Source: three-view drawing plus pictorial views. Frame: mm from the lowest corner of the part. A direction names the side the tool comes from. Coordinates: 2 decimals unless noted, no trailing zeros. Write each loop counter-clockwise with the first axis right and the second up, starting at its lowest first coordinate (ties: lowest second). Pieces come first, ordered by that corner, then holes. Notation, with made-up numbers: (24, -32) - (60, -32) arc R14 cw to (60, -7) - close; hole circle Ø1 at (57, 2). An arc over 180 degrees is marked (long way). One line per item, written item: value.
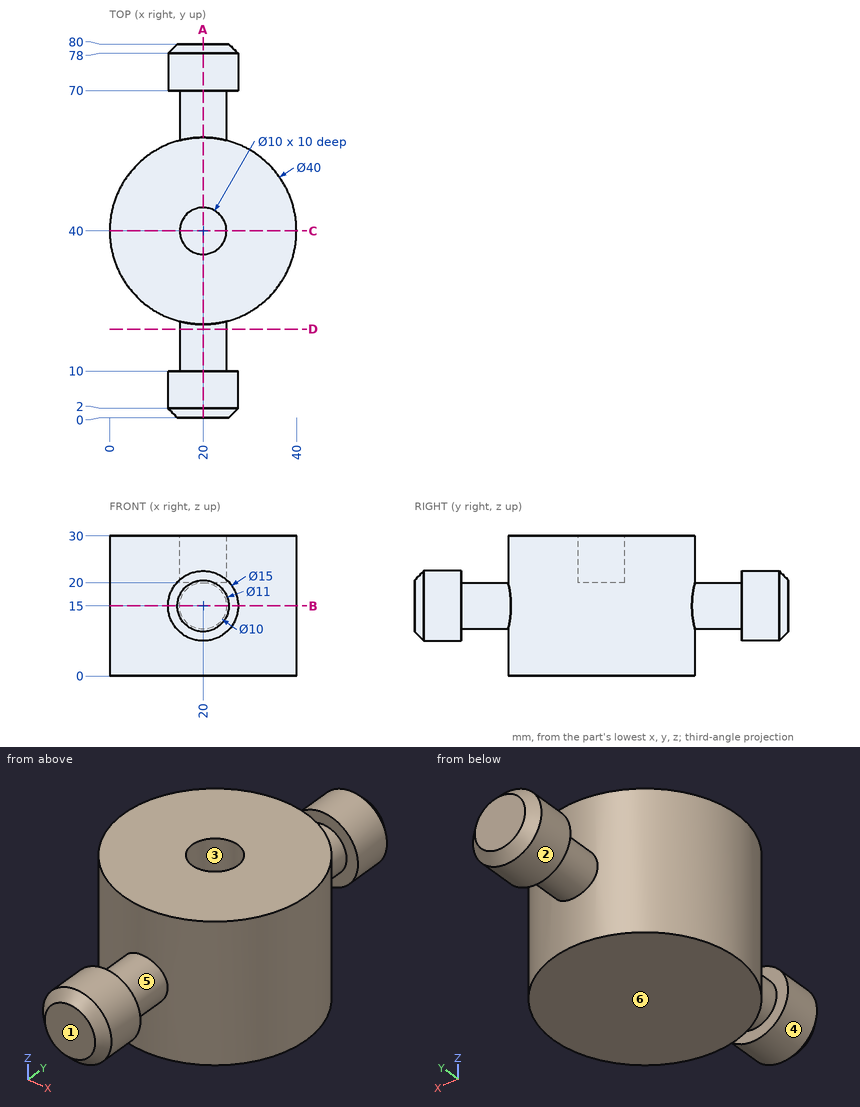
1) Section query B-B on z = 15. Output: boundary loops of the cut face in (x, y).
Values found:
outline: (12.5, 2) - (14.5, 0) - (25.5, 0) - (27.5, 2) - (27.5, 10) - (25, 10) - (25, 20.64) arc R20 ccw to (25, 59.36) - (25, 70) - (27.5, 70) - (27.5, 78) - (25.5, 80) - (14.5, 80) - (12.5, 78) - (12.5, 70) - (15, 70) - (15, 59.36) arc R20 ccw to (15, 20.64) - (15, 10) - (12.5, 10) - close
2) Contact query for flat-ended pins moving along their axis: P1, Ø1, axis at y = 53, z = 8, coming from the +X side; P2, Ø3, axis at x = 32.5, z = 11.5, coming from the +Y side; P3, Ø12, axis at x = 24.5, y = 69, coming from the -Z side. Output: stop coordinate, or through.
Values found:
P1: x = 35.61
P2: y = 56.7
P3: z = 7.5
3) Draft query along Y for the marked faces 1, 2 and 3. Return one class per face: released by +Y, released by -Y, zero draft, split by the parting line, or undercut.
Values found:
face 1: released by -Y
face 2: zero draft
face 3: undercut
4) Section query D-D on y = 19. Output: boundary loops of the cut face in (x, z), then the cut area to 3 significant figures.
Values found:
outline: circle Ø10 at (20, 15)
area: 78.5 mm2
5) Section query C-C on y = 40. Output: boundary loops of the cut face in (x, z).
Values found:
outline: (0, 0) - (40, 0) - (40, 30) - (25, 30) - (25, 20) - (15, 20) - (15, 30) - (0, 30) - close
6) Reachability of the marked faces 4, 5 and 6 from +Z, -Z, +X, -X, +Y, -Y: full face, straight path, thin tool, end or side. Return the list, or none.
Values found:
face 4: -Y
face 5: none
face 6: -Z, +X, -X, +Y, -Y
7) Material intervals for line 1 (Y direction, x = 20, z = 24); line 2 (Y direction, x = 26, z = 18); line 3 (X direction, y = 39.5, z = 3), sorted ascending.
Values found:
line 1: 20 to 35, 45 to 60
line 2: 1.21 to 10, 20.92 to 59.08, 70 to 78.79
line 3: 0.01 to 39.99
8) Section query A-A on x = 20. Output: boundary loops of the cut face in (y, z).
Values found:
outline: (0, 9.5) - (2, 7.5) - (10, 7.5) - (10, 10) - (20, 10) - (20, 0) - (60, 0) - (60, 10) - (70, 10) - (70, 7.5) - (78, 7.5) - (80, 9.5) - (80, 20.5) - (78, 22.5) - (70, 22.5) - (70, 20) - (60, 20) - (60, 30) - (45, 30) - (45, 20) - (35, 20) - (35, 30) - (20, 30) - (20, 20) - (10, 20) - (10, 22.5) - (2, 22.5) - (0, 20.5) - close
